Autodesk Inventor part; units mm, degrees
ref_plane "YZ Plane" through (0, 0, 0) normal (1, 0, 0) x (0, 1, 0)
ref_plane "XZ Plane" through (0, 0, 0) normal (0, 1, 0) x (-1, 0, 0)
ref_plane "XY Plane" through (0, 0, 0) normal (0, 0, 1) x (1, 0, 0)
sketch "Sketch1" plane through (0, 0, 0) normal (0, 0, 1) x (1, 0, 0)
  line L0 (-14.0074, 10.2243) -> (11.3926, 10.2243)
  line L1 (11.3926, 10.2243) -> (11.3926, -15.1757)
  line L2 (11.3926, -15.1757) -> (-14.0074, -15.1757)
  line L3 (-14.0074, -15.1757) -> (-14.0074, 10.2243)
  line L4 (10.1226, 8.9543) -> (-12.7374, 8.9543)
  line L5 (-12.7374, 8.9543) -> (-12.7374, -13.9057)
  line L6 (-12.7374, -13.9057) -> (10.1226, -13.9057)
  line L7 (10.1226, -13.9057) -> (10.1226, 8.9543)
  point P0 (0, 0)
  dimension "d0" = 25.4
  dimension "d1" = 1.27
extrude "Extrusion1" add sketch "Sketch1" along normal blind 711.2
sketch "Sketch2" plane through (11.3926, -15.1757, 0) normal (1, 0, 0) x (0, 0, -1)
  circle A0 centre (-355.6, 12.7) radius 7.9375
  line L0 (-711.2, 1.27) -> (-711.2, 24.13)
  line L1 (-711.2, 12.7) -> (0, 12.7) construction
  line L2 (0, 25.4) -> (0, 0)
  circle A1 centre (-533.4, 12.7) radius 7.9375
  circle A2 centre (-177.8, 12.7) radius 7.9375
  point P0 (0, 15.1757)
  dimension "d5" = 15.875
  dimension "d6" = 177.8
  dimension "d7" = 177.8
  dimension "d8" = 355.6
extrude "Extrusion2" cut sketch "Sketch2" against normal blind 2.54
sketch "Sketch3" plane through (-14.0074, -15.1757, 0) normal (-1, 0, 0) x (0, 0, 1)
  circle A0 centre (177.8, 12.7) radius 7.9375 construction
  circle A1 centre (355.6, 12.7) radius 7.9375 construction
  circle A2 centre (533.4, 12.7) radius 7.9375 construction
  circle A3 centre (177.8, 12.7) radius 2.9972
  circle A4 centre (355.6, 12.7) radius 2.9972
  circle A5 centre (533.4, 12.7) radius 2.9972
  point P0 (0, 15.1757)
  dimension "d11" = 5.9944
extrude "Extrusion3" cut sketch "Sketch3" against normal blind 2.54
equation "\"d6\" = d4"
equation "\"d7\" = d4"
equation "\"d8\" = 0.5 * d2"
equation "\"d4\" = 177.8"
properties part number "1x1 28in WChurro Holes"
Read the model definition and answer for the solid it produces. Units are mm, in the model's axes. A direction names the side the tool comes from. Give positions to 0.01 mm unless a question says otherwise; leave off trailing zeros. Write each loop counter-clockwise with the first axis right and the second up, starting at its lowest first coordinate (ties: lowest second). Pieces come first, ordered by that corner, then holes. Notation, with made-up numbers: (20.5, 1.25) - (66.5, 1.25) arc R18 ccw to (66.5, 34.25) - close; hole circle Ø2 at (43.5, -29). An arc over 180 degrees is marked (long way). Use CSV: the item, a comma, the result in double quotes. Start each with the question number.
(1) Find section B-B (z = 234.5). Give the vertices of the cut face in (x, y), plus the area to 3 significant figures.
(2) Find section A-A (x = -8). Give the vertices of the cut face in (y, z), plus the area to 3 significant figures.
(3) For faces 1 (the cylindrical face through (10.77, -2.13, 363.53)), 2 (the flat face through (10.123, 5, 351)), 3 (the flat face through (-2, -15, 0)), determine the directions among +Z, -Z, +X, -X, +Y, -Y from which every point of the face is accessible in a straight line to the end or side of a thin tool.
(4) Consider line 1 along Y through (x, z) = (-6, 47); line 2 along X through (y, z) = (5, 163.5); line 3 along Y through (x, z) = (10.8, 533.4). Determine where each line is inside the solid, lowest interval first.
(5) Given P1, Ø7, axis at y = -2.48, z = 533.4, coming from the +X side, flat-ended and moving along its own axis, determine where the tip first touches the part or whether it passes through.
(6) Determine the mould class of faces 4 (the flat face through (-1, -15.176, 351)), 5 (the flat face through (-1, -13.906, 351)), 6 (the flat face through (11.393, 6, 351)), 7 (the flat face through (-1, 8.954, 351)) for opening direction Y: +Y half, -Y half, draft (parallel to the pull), parting line (faces both ways), or undercut.
Findings below:
1,outline,"(-14.01, -15.18) - (11.39, -15.18) - (11.39, 10.22) - (-14.01, 10.22) - close; hole (-12.74, -13.91) - (10.12, -13.91) - (10.12, 8.95) - (-12.74, 8.95) - close"
1,area,"123 mm2"
2,outline,"(-15.18, 0) - (-13.91, 0) - (-13.91, 711.2) - (-15.18, 711.2) - close; (8.95, 0) - (10.22, 0) - (10.22, 711.2) - (8.95, 711.2) - close"
2,area,"1,810 mm2"
3,face 1,"+X"
3,face 2,"+Z, -Z"
3,face 3,"-Z, +X, -X, +Y, -Y"
4,line 1,"-15.18 to -13.91, 8.95 to 10.22"
4,line 2,"-14.01 to -12.74, 10.12 to 11.39"
4,line 3,"-15.18 to -10.41, 5.46 to 10.22"
5,P1,"x = -12.74"
6,face 4,"-Y half"
6,face 5,"undercut"
6,face 6,"draft"
6,face 7,"undercut"
